Could you check a few things on this drawing? It's one solid part, dimensions in mm from its lowest x, y, z. Round coordinates to 2 decimals unless told otherwise and drop trailing zeros. Loops run counter-clockwise (first coordinate to the right, second up) from the corner with the lowest first, then second, coordinate; pieces in that order, holes last. Notation, with made-up numbers: (4, -25) -> (32, -25) arc R24 cw to (32, 8) -> close; hole circle Ø4 at (75.5, 49). An arc over 180 degrees is marked (long way). Use one line per item in the form item = value. Start each with the question number.
Item 1: Thinking about a two-plate mould opening in Y: for the marked faces 1 and 2, which applies, released by +Y, released by -Y, zero draft, split by the parting line, or undercut?
Item 2: If I drill on L1, parallel to Y at x = 21, z = 40.5; L2, parallel to X at y = 8, z = 40; L3, parallel to X at y = 18.5, z = 43, over which ranges is the centre line in solid material (lowest first)? Write a range as [from, to].
Item 3: If we section it at C-C (z = 151.5): Write out the boundary of the cut face in (x, y).
Item 4: I'm going to push flat-ended pins straight in: pin 1 Ø8 at (x, z) = (26.5, 133) entering from -Y; pin 2 Ø1.5 at (y, z) = (26.5, 66) entering from -X; pin 3 Ø4 at (y, z) = (14.5, 129) entering from +X; pin 4 Ø10 at (x, y) = (30, 27.5) entering from +Z. Where does each tip first touch, or does it pass through?
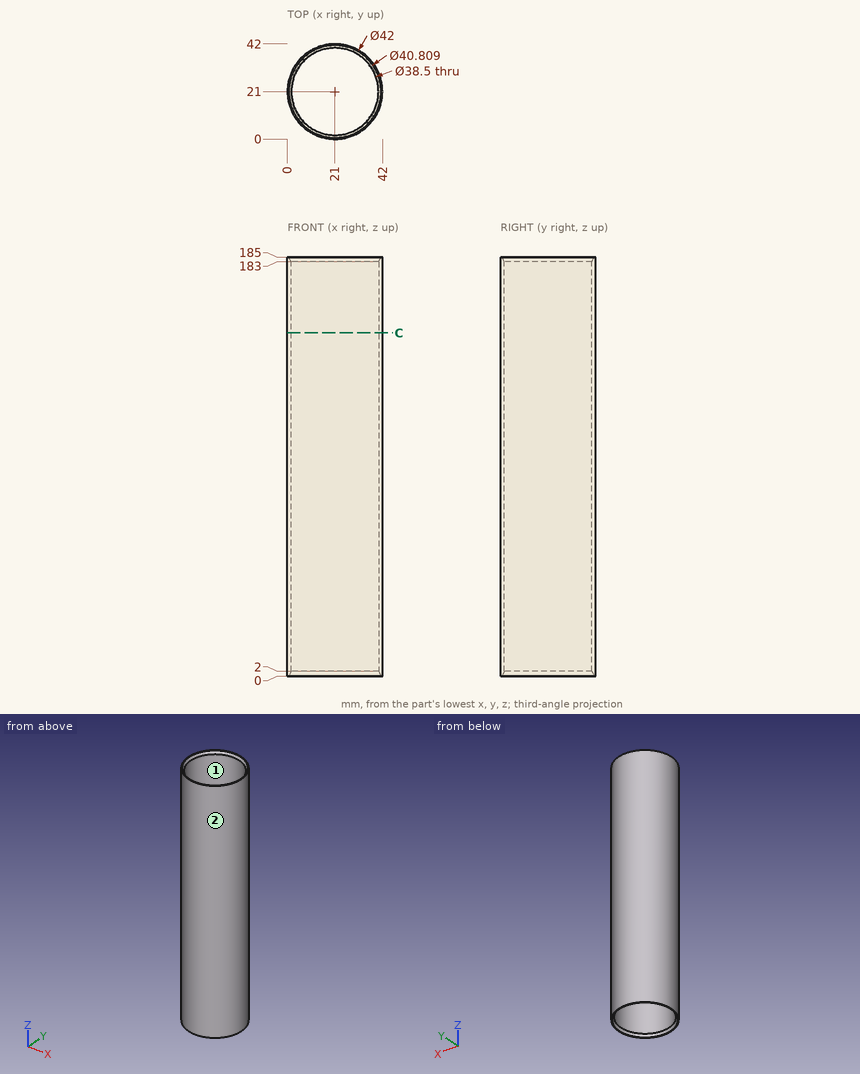
Values found:
q1.face_1 = undercut
q1.face_2 = split by the parting line
q2.L1 = [0, 1.75], [40.25, 42]
q2.L2 = [4.51, 6.8], [35.2, 37.49]
q2.L3 = [0.15, 1.91], [40.09, 41.85]
q3.outline = circle Ø42 at (21, 21); hole circle Ø38.5 at (21, 21)
q4.pin_1 = 0.05
q4.pin_2 = 0.54
q4.pin_3 = 41.51
q4.pin_4 = through
